```python
from build123d import *

# Parameters (mm, degrees)
F1_DEPTH = 15
F2_R     = 4.99999
F3_R     = 2.5
F4_DEPTH = 15.001


# Not quite as in the source:
# - a fillet or chamfer is up to 0.001 mm smaller than in the source, because OpenCascade refuses the exact size


with BuildPart() as f1:
    # F0 (on Front) → F1 (new body)
    with BuildSketch(Plane.XZ):
        with BuildLine():
            Line((-15, 40), (-15, 20))
            ThreePointArc((-15, 20), (-23.7170824513, -7.9056941504), (0, -25))
            Line((0, -25), (0, -15))
            ThreePointArc((0, -15), (-14.7839783948, -2.5365296809), (-5, 14.1421356237))
            Line((-5, 14.1421356237), (-5, 40))
            Line((-5, 40), (-15, 40))
        make_face()
    extrude(amount=F1_DEPTH)

    # F2 (radius 5 in the source; OpenCascade refuses exactly that, so slightly less here)
    f2_edges = [f1.edges().sort_by_distance(p)[0] for p in [
        (0, -7.5, -25),
        (0, -7.5, -15),
    ]]
    fillet(f2_edges, radius=F2_R)

    # F3 (on face) → F4 (cut, through all)
    with BuildSketch(Plane.XZ.offset(15)):
        with Locations((-5, -19.364916731)):
            Circle(F3_R)
    extrude(amount=-F4_DEPTH, mode=Mode.SUBTRACT)


solid = f1.part
```
Could you check a few things on this model? Use its own coordinates, in mm. A direction names the side the tool comes from. Coordinates: 2 decimals unless noted, no trailing zeros. Write each loop counter-clockwise with the first axis right and the second up, starting at its lowest first coordinate (ties: lowest second). Pieces come first, ordered by that corner, then holes. Notation, with made-up numbers: (-8, -17) -> (6, -17) arc R25 ccw to (6, 12) -> close; hole circle Ø10 at (48, -29). An arc over 180 degrees is marked (long way). Return JSON: item names as keys, results as strings.
(1) I'm going to push flat-ended pins straight in: pin 1 (5 mm diameter, centred on y = -7.5, z = 5, fed in from -X); pin 2 (3 mm diameter, centred on y = -13.5, z = -11.5, fed in from -X); pin 3 (6 mm diameter, centred on y = -5, z = 18.5, fed in from +X). Where does each tip first touch, or does it pass through?
Numbers:
{"pin 1": "stops at x = -24.87", "pin 2": "stops at x = -22.91", "pin 3": "stops at x = -5"}
(2) Imagine slicing it at B-B, the plane x = -12.5. Please give me the cut outline in (y, z).
Numbers:
{"outline": "(-15, -21.65) -> (0, -21.65) -> (0, -8.29) -> (-15, -8.29) -> close; (-15, 8.29) -> (0, 8.29) -> (0, 40) -> (-15, 40) -> close"}
(3) Imagine slicing it at D-D, the plane x = -19.25. Please give me the cut outline in (y, z), then the cut area to 3 significant figures.
Numbers:
{"outline": "(-15, -15.95) -> (0, -15.95) -> (0, 15.95) -> (-15, 15.95) -> close", "area": "479 mm2"}
(4) I need wall thicknesses on L1, parallel to Z at x = -6, y = -2.75; L2, parallel to X at y = -5.5, z = 33; L3, parallel to X at y = -5.25, z = 0. Which ranges of each line are inside material? Lowest first, please.
Numbers:
{"L1": "z = -24.26 to -21.66, -17.07 to -13.75, 13.75 to 40", "L2": "x = -15 to -5", "L3": "x = -25 to -15"}
(5) Imagine slicing it at C-C, the plane z = 22.5. Please give me the cut outline in (x, y), then the cut area to 3 significant figures.
Numbers:
{"outline": "(-15, -15) -> (-5, -15) -> (-5, 0) -> (-15, 0) -> close", "area": "150 mm2"}
(6) We'd pull the mould along Z, two halves only. Please class faces 1 (the cylindrical face through (-1.02, -7.6, -16.34)), 2 (the flat face through (-5, -7, 27)), 3 (the cylindrical face through (-3.656, -7.605, -17.257)): +Z half, -Z half, draft (parallel to the pull), parting line (faces both ways), or undercut.
Numbers:
{"face 1": "+Z half", "face 2": "draft", "face 3": "undercut"}
(7) Which directions (+Z, -Z, +X, -X, +Y, -Y) give clear straight access to the entire face, cutting with the end or side of a thin tool? Please do faces 4 (the flat face through (-15, -7, 30)), 5 (the cylindrical face through (-14.97, -7.4, -0.92)).
Numbers:
{"face 4": "+Z, -X, +Y, -Y", "face 5": "+X, +Y, -Y"}
